```python
from build123d import *

# Parameters (mm, degrees)
SKETCH_4_W          = 57
SKETCH_4_H          = 145
EXTRUDE_1_DEPTH     = 4
SKETCH_5_W          = 7.875
SKETCH_5_H          = 4
EXTRUDE_2_DEPTH     = 2
SKETCH_6_W          = 21
SKETCH_6_H          = 4
EXTRUDE_3_DEPTH     = 2
EXTRUDE_START       = -57
SKETCH_6_2_W        = 21
SKETCH_6_2_H        = 4
EXTRUDE_4_DEPTH     = 4
CUT_EXTRUDE_START   = -1.8
SKETCH_7_W          = 10.3
SKETCH_7_H          = 2.2
CUT_EXTRUDE_1_DEPTH = 149.802954818
CUT_EXTRUDE_2_DEPTH = 82.310146968


with BuildPart() as part:
    # 草图4 → 凸台-拉伸1 (new body)
    with BuildSketch(Plane(origin=(0, 0, 0), x_dir=(1, 0, 0), z_dir=(0, 1, 0))):
        Rectangle(SKETCH_4_W, SKETCH_4_H)
    extrude(amount=EXTRUDE_1_DEPTH)

    # 草图5 → 凸台-拉伸2 (add)
    with BuildSketch(Plane(origin=(0, 0, -72.5), x_dir=(-1, 0, 0), z_dir=(0, 0, -1))):
        with Locations((-24.5625, 2)):
            Rectangle(SKETCH_5_W, SKETCH_5_H)
        with Locations((-8.1875, 2)):
            Rectangle(SKETCH_5_W, SKETCH_5_H)
        with Locations((8.1875, 2)):
            Rectangle(SKETCH_5_W, SKETCH_5_H)
        with Locations((24.5625, 2)):
            Rectangle(SKETCH_5_W, SKETCH_5_H)
    extrude(amount=EXTRUDE_2_DEPTH)

    # 草图6 → 凸台-拉伸3 (add)
    with BuildSketch(Plane.ZY.offset(28.5)):
        with Locations((-43, 2)):
            Rectangle(SKETCH_6_W, SKETCH_6_H)
        with Locations((-1, 2)):
            Rectangle(SKETCH_6_W, SKETCH_6_H)
        with Locations((41, 2)):
            Rectangle(SKETCH_6_W, SKETCH_6_H)
    extrude(amount=EXTRUDE_3_DEPTH)

    # 草图6<2> → 凸台-拉伸4 (add)
    with BuildSketch(Plane.ZY.offset(28.5).offset(EXTRUDE_START)):
        with Locations((-43, 2)):
            Rectangle(SKETCH_6_2_W, SKETCH_6_2_H)
        with Locations((-1, 2)):
            Rectangle(SKETCH_6_2_W, SKETCH_6_2_H)
        with Locations((41, 2)):
            Rectangle(SKETCH_6_2_W, SKETCH_6_2_H)
    extrude(amount=-EXTRUDE_4_DEPTH)

    # 草图7 → 切除-拉伸1 (cut, through all)
    with BuildSketch(Plane.XY.offset(72.5).offset(CUT_EXTRUDE_START)):
        Polygon((-10.3, 2.2), (-10.3, 0), (-12.5, 2.2), align=None)
        with Locations((-5.15, 1.1)):
            Rectangle(SKETCH_7_W, SKETCH_7_H)
        with Locations((5.15, 1.1)):
            Rectangle(SKETCH_7_W, SKETCH_7_H)
        Polygon((10.3, 2.2), (12.5, 2.2), (10.3, 0), align=None)
    extrude(amount=-CUT_EXTRUDE_1_DEPTH, mode=Mode.SUBTRACT)

    # 草图8 → 切除-拉伸2 (cut, through all)
    with BuildSketch(Plane.XZ.offset(-2.2)):
        Polygon((-12.5, -61.018518519), (-16.375, -72.5), (-12.5, -72.5), align=None)
        Polygon((-10.3, -54.5), (-12.5, -61.018518519), (-12.5, -72.5), (-12.125, -72.5), (-4.25, -72.5), (4.25, -72.5), (12.125, -72.5), (12.5, -72.5), (12.5, -61.018518519), (10.3, -54.5), align=None)
        Polygon((12.5, -72.5), (16.375, -72.5), (12.5, -61.018518519), align=None)
    extrude(amount=CUT_EXTRUDE_2_DEPTH, mode=Mode.SUBTRACT)


with BuildPart() as cut_extrude_2_kept_piece:
    # of the separate pieces the step leaves, the one the design keeps (cut_extrude_2_pieces_kept)
    add(part.part.solids().sort_by_distance((-28.5, 0, 72.5))[0])


solid = cut_extrude_2_kept_piece.part
```
Geometry check sheet. Reference: the model listing, model coordinates, mm. A direction names the side the tool comes from. Round coordinates to 2 decimals unless told otherwise and drop trailing zeros. Write each loop counter-clockwise with the first axis right and the second up, starting at its lowest first coordinate (ties: lowest second). Pieces come first, ordered by that corner, then holes. Notation, with made-up numbers: (6.25, 72) -> (12.25, 72) arc R34 ccw to (12.25, 111) -> close; hole circle Ø7 at (-15.75, 43). An arc over 180 degrees is marked (long way). Put each result on its own line as item: value.
1) Cross-section at C-C, the plane z = 3. Enter the section's corners in (x, y), plus the area to 3 significant figures.
Recorded:
outline: (-30.5, 0) -> (-10.3, 0) -> (-12.5, 2.2) -> (12.5, 2.2) -> (10.3, 0) -> (32.5, 0) -> (32.5, 4) -> (-30.5, 4) -> close
area: 202 mm2
2) Depth check by flat-ended pin: P1, Ø0.6, axis at x = -30, y = 2, coming from the -Z side; P2, Ø1.2, axis at x = 15, y = 2, coming from the -Z side; P3, Ø2, axis at y = 2, z = -73.5, coming from the +X side. Enter the tip coordinate at first touch or a pass-through.
Recorded:
P1: stops at z = -53.5
P2: stops at z = -72.5
P3: stops at x = 28.5
3) Release check for a two-part mould opening along Z. For faces 5 (the face through (0, 2.2, -1)), 6 (the face through (30, 2, -53.5)), 7 (the face through (30, 2, 30.5)) record: pulls with the +Z half, pulls with the -Z half, needs draft (parallel to the pull), parting line crosses it, or undercut.
Recorded:
face 5: needs draft
face 6: pulls with the -Z half
face 7: undercut
4) Cross-section at A-A, the plane z = -26.5. Enter the section's corners in (x, y), plus the area to 3 significant figures.
Recorded:
outline: (-28.5, 0) -> (-10.3, 0) -> (-12.5, 2.2) -> (12.5, 2.2) -> (10.3, 0) -> (28.5, 0) -> (28.5, 4) -> (-28.5, 4) -> close
area: 178 mm2
5) Cross-section at B-B, the plane x = -2. Enter the section's corners in (y, z).
Recorded:
outline: (0, 70.7) -> (2.2, 70.7) -> (2.2, -72.5) -> (4, -72.5) -> (4, 72.5) -> (0, 72.5) -> close
6) Cross-section at D-D, the plane z = -56.5. Enter the section's corners in (x, y) (3 decimals), plus the area to 3 significant figures.
Recorded:
outline: (-28.5, 0) -> (-10.975, 0) -> (-10.975, 0.675) -> (-12.5, 2.2) -> (12.5, 2.2) -> (10.975, 0.675) -> (10.975, 0) -> (28.5, 0) -> (28.5, 4) -> (-28.5, 4) -> close
area: 177 mm2
7) Thickness scan on probe 1 along X at (y, z) = (1.8, -3); probe 2 along Z at (x, y) = (19, 0.65); probe 3 along Z at (x, y) = (-5, 1.65). Record the ranges inside material, lowest first. Write a range as from..to.
Recorded:
probe 1: x = -30.5..-12.1, 12.1..32.5
probe 2: z = -72.5..72.5
probe 3: z = 70.7..72.5
8) Access from +Z, -Z, +X, -X, +Y, -Y to the whole of each face (thin tool, end or side, straight path). Record for faces 1 (the face through (28.5, 2, 62)), 2 (the face through (-28.5, 2, 62)), 3 (the face through (30, 2, -11.5)), 4 (the face through (-28.5, 2, -22)).
Recorded:
face 1: +Z, +X, +Y, -Y
face 2: +Z, -X, +Y, -Y
face 3: +X, +Y, -Y
face 4: -X, +Y, -Y
